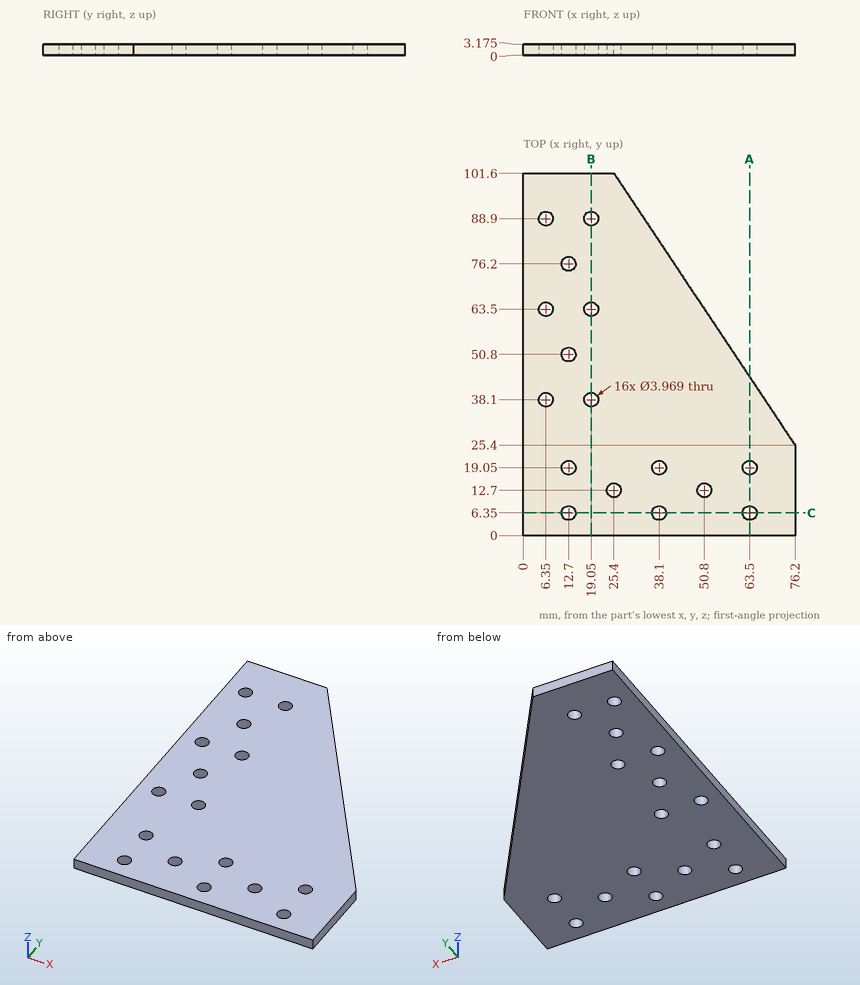
For this review, use the dimensioned drawing (mm, ordinates from the lowest corner) and the shaded views. Give positions to 0.01 mm unless a question says otherwise; leave off trailing zeros. Order: outer loops, then holes, each group sorted by start corner. A loop starts at its lowest first (then second) coordinate and runs counter-clockwise, first axis right, second up. Notation, with made-up numbers: M 38.25,9 L 54.25,9 A29 cw 54.25,41 Z; hole C 85.5,31 d3. An arc over 180 degrees is marked long. One line per question, with ' | ' between items. Start each with the question number.
1) Consider section A-A, the plane x = 63.5. State how many separate pieces and enclosed holes the cut face has, then the cut area to 3 significant figures.
2) Consider section B-B, the plane x = 19.05. Give the boundary of the cut face in (y, z) (1 decimal), then the cut area to 3 significant figures.
3) Wall thickness on L1, parallel to Y at x = 12.5, z = 2.7; L2, parallel to X at y = 12.7, z = 0.7; L3, parallel to X at y = 63.5, z = 1.35 (1 decimal): over which ranges is each line inside the solid? List them lowest first. Write a range as from..to.
4) Consider section C-C, the plane y = 6.35. Give the boundary of the cut face in (x, z) (1 decimal), then the cut area to 3 significant figures.
5) Clearance check with a flat-ended pin moving along its axis: P1, Ø3, axis at x = 12.7, y = 76.2, coming from the +Z side. State where the tip first meets the part, or that it passes through.
Found:
1) separate pieces: 3 | enclosed holes: 0 | area: 116 mm²
2) outline: M 0,0 L 36.1,0 L 36.1,3.2 L 0,3.2 Z; M 40.1,0 L 61.5,0 L 61.5,3.2 L 40.1,3.2 Z; M 65.5,0 L 86.9,0 L 86.9,3.2 L 65.5,3.2 Z; M 90.9,0 L 101.6,0 L 101.6,3.2 L 90.9,3.2 Z | area: 285 mm²
3) L1: y = 0..4.38, 8.32..17.08, 21.02..48.83, 52.77..74.23, 78.17..101.6 | L2: x = 0..23.42, 27.38..48.82, 52.78..76.2 | L3: x = 0..4.4, 8.3..17.1, 21..50.8
4) outline: M 0,0 L 10.7,0 L 10.7,3.2 L 0,3.2 Z; M 14.7,0 L 36.1,0 L 36.1,3.2 L 14.7,3.2 Z; M 40.1,0 L 61.5,0 L 61.5,3.2 L 40.1,3.2 Z; M 65.5,0 L 76.2,0 L 76.2,3.2 L 65.5,3.2 Z | area: 204 mm²
5) P1: passes through
